For this review, take the finished solid that the model builds, in its own axes (mm). A direction names the side the tool comes from. Coordinates: 2 decimals unless noted, no trailing zeros. Write each loop counter-clockwise with the first axis right and the second up, starting at its lowest first coordinate (ties: lowest second). Pieces come first, ordered by that corner, then holes.
```python
from build123d import *

# Parameters (mm, degrees)
SKETCH_1_R               = 25
EXTRUDE_1_DEPTH          = 30
SKETCH_2_R               = 25
EXTRUDE_2_DEPTH          = 250
SKETCH_3_W               = 40
SKETCH_3_H               = 10
EXTRUDE_4_DEPTH          = 40
CUT_EXTRUDE_1_DEPTH      = 323.877685819
CUT_EXTRUDE_1_DEPTH_BACK = 323.877685819
CUT_EXTRUDE_2_DEPTH      = 323.877685819
CUT_EXTRUDE_2_DEPTH_BACK = 323.877685819
SKETCH_7_R               = 10


with BuildPart() as part:
    # 스케치1 → 보스-돌출1 (new body)
    with BuildSketch(Plane.XY):
        Circle(SKETCH_1_R)
    extrude(amount=-EXTRUDE_1_DEPTH)

    # 스케치2 → 보스-돌출2 (add)
    with BuildSketch(Plane(origin=(0, 0, -30), x_dir=(-1, 0, 0), z_dir=(0, 0, -1))):
        with Locations(Location((0, 0, 0), (0, 0, 180))):
            Circle(SKETCH_2_R)
    extrude(amount=EXTRUDE_2_DEPTH)

    # 스케치3 → 보스-돌출4 (add)
    with BuildSketch(Plane(origin=(0, 0, -280), x_dir=(-1, 0, 0), z_dir=(0, 0, -1))):
        with Locations((0, -5)):
            Rectangle(SKETCH_3_W, SKETCH_3_H)
        with Locations((0, 5)):
            Rectangle(SKETCH_3_W, SKETCH_3_H)
    extrude(amount=EXTRUDE_4_DEPTH)

    # 스케치6 → 컷-돌출1 (cut, two sides: drawn at the far end of the back side and taken through both)
    with BuildSketch(Plane(origin=(0, 10, 0), x_dir=(1, 0, 0), z_dir=(0, 1, 0)).offset(-CUT_EXTRUDE_1_DEPTH_BACK)):
        with BuildLine():
            ThreePointArc((-20, 300), (-14.142135624, 314.142135624), (0, 320))
            Line((0, 320), (-20, 320))
            Line((-20, 320), (-20, 300))
        make_face()
        with BuildLine():
            Line((20, 320), (0, 320))
            ThreePointArc((0, 320), (14.142135624, 314.142135624), (20, 300))
            Line((20, 300), (20, 320))
        make_face()
    extrude(amount=CUT_EXTRUDE_1_DEPTH + CUT_EXTRUDE_1_DEPTH_BACK, mode=Mode.SUBTRACT)

    # 스케치7 → 컷-돌출2 (cut, two sides: drawn at the far end of the back side and taken through both)
    with BuildSketch(Plane(origin=(0, 10, 0), x_dir=(1, 0, 0), z_dir=(0, 1, 0)).offset(-CUT_EXTRUDE_2_DEPTH_BACK)):
        with Locations(Location((0, 300, 0), (0, 0, 270))):
            Circle(SKETCH_7_R)
    extrude(amount=CUT_EXTRUDE_2_DEPTH + CUT_EXTRUDE_2_DEPTH_BACK, mode=Mode.SUBTRACT)


solid = part.part
```
1) Consider section A-A (y = 0). Give the boundary of the cut face in (x, z), then the cut area to 3 significant figures.
2) The part is to be moulded in two halves that separate along X. For faces 1 (the face through (0, 11, -280)), 2 (the face through (0, 0, -310)), 3 (the face through (23.846, -7.509, -138.04)), 4 (the face through (20, 0, -290)), say which applies: pulls with the +X half, pulls with the -X half, needs draft (parallel to the pull), parting line crosses it, or undercut.
3) Consider section D-D (z = -84). Give the boundary of the cut face in (x, y), then the cut area to 3 significant figures.
4) For L1, parallel to X at y = 0, z = -300; L2, parallel to Z at x = -1, y = 5; L3, parallel to Y at x = 0.5, z = -72 (3 decimals), list the stretches that pass through material, from the lowest coordinate up.
5) Consider section B-B (x = -3.5). Give the boundary of the cut face in (y, z), then the cut area to 3 significant figures.
6) Clearance check with flat-ended pins moving along their axes: P1, Ø6, axis at y = -4, z = -290.5, coming from the +X side; P2, Ø5, axis at x = -7, y = 12, coming from the -Z side; P3, Ø5, axis at x = -17.5, z = -273.5, coming from the +Y side; P4, Ø8, axis at x = -3.5, y = 11.5, coming from the +Z side. State where each tip first meets the part, or that it passes through.
7) Consider section C-C (x = 17). Give the boundary of the cut face in (y, z), then the cut area to 3 significant figures.
8) Tool access review of faces 5 (the face through (-20, 0, -290)), 6 (the face through (5, -10, -291)), 7 (the face through (5, 10, -291)): name each direction out of +Z, -Z, +X, -X, +Y, -Y from which nothing blocks a thin tool from reaching the whole face with its end or side.
Results:
1. outline: (-25, -280) - (-20, -280) - (-20, -300) arc R20 ccw to (20, -300) - (20, -280) - (25, -280) - (25, 0) - (-25, 0) - close; hole circle Ø20 at (0, -300)
1. area: 15,100 mm2
2. face 1: needs draft
2. face 2: undercut
2. face 3: parting line crosses it
2. face 4: pulls with the +X half
3. outline: circle Ø50 at (0, 0)
3. area: 1,960 mm2
4. L1: x = -20 to -10, 10 to 20
4. L2: z = -319.97 to -309.95, -290.05 to 0
4. L3: y = -24.995 to 24.995
5. outline: (-24.75, -280) - (-10, -280) - (-10, -290.63) - (10, -290.63) - (10, -280) - (24.75, -280) - (24.75, 0) - (-24.75, 0) - close; (-10, -319.69) - (10, -319.69) - (10, -309.37) - (-10, -309.37) - close
5. area: 14,300 mm2
6. P1: stops at x = 20
6. P2: stops at z = -319.23
6. P3: stops at y = 20
6. P4: stops at z = 0
7. outline: (-18.33, -280) - (-10, -280) - (-10, -310.54) - (10, -310.54) - (10, -280) - (18.33, -280) - (18.33, 0) - (-18.33, 0) - close
7. area: 10,900 mm2
8. face 5: -Z, -X, +Y, -Y
8. face 6: -Z, +X, -X, -Y
8. face 7: -Z, +X, -X, +Y
